Can you work these out from the model? Positions are in its coordinate system, mm. Give positions to 0.01 mm unless a question says otherwise; leave off trailing zeros. Write each loop counter-clockwise with the first axis right and the second up, starting at its lowest first coordinate (ties: lowest second). Pieces come first, ordered by that corner, then holes. Notation, with made-up numbers: (-11.5, 49) -> (45.5, 49) arc R27 cw to (45.5, 72) -> close; hole circle Ø4 at (-21.75, 54). An arc over 180 degrees is marked (long way). One line per item, written item: value.
from build123d import *

# Parameters (mm, degrees)
F0_W     = 508
F0_H     = 127
F0_R     = 9.525
F1_DEPTH = 25.4
F3_DEPTH = 101.6


# Not quite as in the source:
# - a fillet or chamfer that OpenCascade refuses, or shapes differently, is made with other operations: its cross-section is extruded or revolved along the edge and cut away or added


with BuildPart() as f1:
    # F0 (on Top) → F1 (new body)
    with BuildSketch(Plane.XY):
        with Locations((254, 63.5)):
            Rectangle(F0_W, F0_H)
        with Locations((63.5, 50.8)):
            Circle(F0_R, mode=Mode.SUBTRACT)
        with Locations((190.5, 50.8)):
            Circle(F0_R, mode=Mode.SUBTRACT)
        with Locations((317.5, 50.8)):
            Circle(F0_R, mode=Mode.SUBTRACT)
        with Locations((444.5, 50.8)):
            Circle(F0_R, mode=Mode.SUBTRACT)
        with Locations((63.5, 76.2)):
            Circle(F0_R, mode=Mode.SUBTRACT)
        with Locations((190.5, 76.2)):
            Circle(F0_R, mode=Mode.SUBTRACT)
        with Locations((317.5, 76.2)):
            Circle(F0_R, mode=Mode.SUBTRACT)
        with Locations((444.5, 76.2)):
            Circle(F0_R, mode=Mode.SUBTRACT)
    extrude(amount=F1_DEPTH)

    # F2: fillet of radius 5.08 on 16 edges, made by hand

    # F2_s1 → F2_t2 (revolve, cut)
    with BuildSketch(Plane.XZ.offset(-76.2)):
        with BuildLine():
            ThreePointArc((200.025, 20.32), (201.5128975516, 23.9121024484), (205.105, 25.4))
            Line((205.105, 25.4), (200.025, 25.4))
            Line((200.025, 25.4), (200.025, 20.32))
        make_face()
    revolve(axis=Axis((190.5, 76.2, 25.4), (0, 0, 1)), mode=Mode.SUBTRACT)

    # F2_s3 → F2_t4 (revolve, cut)
    with BuildSketch(Plane.XZ.offset(-50.8)):
        with BuildLine():
            ThreePointArc((200.025, 20.32), (201.5128975516, 23.9121024484), (205.105, 25.4))
            Line((205.105, 25.4), (200.025, 25.4))
            Line((200.025, 25.4), (200.025, 20.32))
        make_face()
    revolve(axis=Axis((190.5, 50.8, 25.4), (0, 0, 1)), mode=Mode.SUBTRACT)

    # F2_s5 → F2_t6 (revolve, cut)
    with BuildSketch(Plane.XZ.offset(-76.2)):
        with BuildLine():
            ThreePointArc((327.025, 20.32), (328.5128975516, 23.9121024484), (332.105, 25.4))
            Line((332.105, 25.4), (327.025, 25.4))
            Line((327.025, 25.4), (327.025, 20.32))
        make_face()
    revolve(axis=Axis((317.5, 76.2, 25.4), (0, 0, 1)), mode=Mode.SUBTRACT)

    # F2_s7 → F2_t8 (revolve, cut)
    with BuildSketch(Plane.XZ.offset(-50.8)):
        with BuildLine():
            ThreePointArc((327.025, 20.32), (328.5128975516, 23.9121024484), (332.105, 25.4))
            Line((332.105, 25.4), (327.025, 25.4))
            Line((327.025, 25.4), (327.025, 20.32))
        make_face()
    revolve(axis=Axis((317.5, 50.8, 25.4), (0, 0, 1)), mode=Mode.SUBTRACT)

    # F2_s9 → F2_t10 (revolve, cut)
    with BuildSketch(Plane.XZ.offset(-76.2)):
        with BuildLine():
            ThreePointArc((73.025, 20.32), (74.5128975516, 23.9121024484), (78.105, 25.4))
            Line((78.105, 25.4), (73.025, 25.4))
            Line((73.025, 25.4), (73.025, 20.32))
        make_face()
    revolve(axis=Axis((63.5, 76.2, 25.4), (0, 0, 1)), mode=Mode.SUBTRACT)

    # F2_s11 → F2_t12 (revolve, cut)
    with BuildSketch(Plane.XZ.offset(-50.8)):
        with BuildLine():
            ThreePointArc((73.025, 20.32), (74.5128975516, 23.9121024484), (78.105, 25.4))
            Line((78.105, 25.4), (73.025, 25.4))
            Line((73.025, 25.4), (73.025, 20.32))
        make_face()
    revolve(axis=Axis((63.5, 50.8, 25.4), (0, 0, 1)), mode=Mode.SUBTRACT)

    # F2_s13 → F2_t14 (revolve, cut)
    with BuildSketch(Plane.XZ.offset(-76.2)):
        with BuildLine():
            ThreePointArc((454.025, 20.32), (455.5128975516, 23.9121024484), (459.105, 25.4))
            Line((459.105, 25.4), (454.025, 25.4))
            Line((454.025, 25.4), (454.025, 20.32))
        make_face()
    revolve(axis=Axis((444.5, 76.2, 25.4), (0, 0, 1)), mode=Mode.SUBTRACT)

    # F2_s15 → F2_t16 (revolve, cut)
    with BuildSketch(Plane.XZ.offset(-50.8)):
        with BuildLine():
            ThreePointArc((454.025, 20.32), (455.5128975516, 23.9121024484), (459.105, 25.4))
            Line((459.105, 25.4), (454.025, 25.4))
            Line((454.025, 25.4), (454.025, 20.32))
        make_face()
    revolve(axis=Axis((444.5, 50.8, 25.4), (0, 0, 1)), mode=Mode.SUBTRACT)

    # F2_s17 → F2_t18 (revolve, cut)
    with BuildSketch(Plane.XZ.offset(-50.8)):
        with BuildLine():
            ThreePointArc((200.025, 5.08), (201.5128975516, 1.4878975516), (205.105, 0))
            Line((205.105, 0), (200.025, 0))
            Line((200.025, 0), (200.025, 5.08))
        make_face()
    revolve(axis=Axis((190.5, 50.8, 0), (0, 0, 1)), mode=Mode.SUBTRACT)

    # F2_s19 → F2_t20 (revolve, cut)
    with BuildSketch(Plane.XZ.offset(-76.2)):
        with BuildLine():
            ThreePointArc((200.025, 5.08), (201.5128975516, 1.4878975516), (205.105, 0))
            Line((205.105, 0), (200.025, 0))
            Line((200.025, 0), (200.025, 5.08))
        make_face()
    revolve(axis=Axis((190.5, 76.2, 0), (0, 0, 1)), mode=Mode.SUBTRACT)

    # F2_s21 → F2_t22 (revolve, cut)
    with BuildSketch(Plane.XZ.offset(-50.8)):
        with BuildLine():
            ThreePointArc((327.025, 5.08), (328.5128975516, 1.4878975516), (332.105, 0))
            Line((332.105, 0), (327.025, 0))
            Line((327.025, 0), (327.025, 5.08))
        make_face()
    revolve(axis=Axis((317.5, 50.8, 0), (0, 0, 1)), mode=Mode.SUBTRACT)

    # F2_s23 → F2_t24 (revolve, cut)
    with BuildSketch(Plane.XZ.offset(-76.2)):
        with BuildLine():
            ThreePointArc((327.025, 5.08), (328.5128975516, 1.4878975516), (332.105, 0))
            Line((332.105, 0), (327.025, 0))
            Line((327.025, 0), (327.025, 5.08))
        make_face()
    revolve(axis=Axis((317.5, 76.2, 0), (0, 0, 1)), mode=Mode.SUBTRACT)

    # F2_s25 → F2_t26 (revolve, cut)
    with BuildSketch(Plane.XZ.offset(-50.8)):
        with BuildLine():
            ThreePointArc((454.025, 5.08), (455.5128975516, 1.4878975516), (459.105, 0))
            Line((459.105, 0), (454.025, 0))
            Line((454.025, 0), (454.025, 5.08))
        make_face()
    revolve(axis=Axis((444.5, 50.8, 0), (0, 0, 1)), mode=Mode.SUBTRACT)

    # F2_s27 → F2_t28 (revolve, cut)
    with BuildSketch(Plane.XZ.offset(-76.2)):
        with BuildLine():
            ThreePointArc((454.025, 5.08), (455.5128975516, 1.4878975516), (459.105, 0))
            Line((459.105, 0), (454.025, 0))
            Line((454.025, 0), (454.025, 5.08))
        make_face()
    revolve(axis=Axis((444.5, 76.2, 0), (0, 0, 1)), mode=Mode.SUBTRACT)

    # F2_s29 → F2_t30 (revolve, cut)
    with BuildSketch(Plane.XZ.offset(-76.2)):
        with BuildLine():
            ThreePointArc((73.025, 5.08), (74.5128975516, 1.4878975516), (78.105, 0))
            Line((78.105, 0), (73.025, 0))
            Line((73.025, 0), (73.025, 5.08))
        make_face()
    revolve(axis=Axis((63.5, 76.2, 0), (0, 0, 1)), mode=Mode.SUBTRACT)

    # F2_s31 → F2_t32 (revolve, cut)
    with BuildSketch(Plane.XZ.offset(-50.8)):
        with BuildLine():
            ThreePointArc((73.025, 5.08), (74.5128975516, 1.4878975516), (78.105, 0))
            Line((78.105, 0), (73.025, 0))
            Line((73.025, 0), (73.025, 5.08))
        make_face()
    revolve(axis=Axis((63.5, 50.8, 0), (0, 0, 1)), mode=Mode.SUBTRACT)

    # F0 (on Top) → F3 (join)
    with BuildSketch(Plane.XY):
        with Locations((254, 63.5)):
            Rectangle(F0_W, F0_H)
        with Locations((63.5, 50.8)):
            Circle(F0_R, mode=Mode.SUBTRACT)
        with Locations((190.5, 50.8)):
            Circle(F0_R, mode=Mode.SUBTRACT)
        with Locations((317.5, 50.8)):
            Circle(F0_R, mode=Mode.SUBTRACT)
        with Locations((444.5, 50.8)):
            Circle(F0_R, mode=Mode.SUBTRACT)
        with Locations((63.5, 76.2)):
            Circle(F0_R, mode=Mode.SUBTRACT)
        with Locations((190.5, 76.2)):
            Circle(F0_R, mode=Mode.SUBTRACT)
        with Locations((317.5, 76.2)):
            Circle(F0_R, mode=Mode.SUBTRACT)
        with Locations((444.5, 76.2)):
            Circle(F0_R, mode=Mode.SUBTRACT)
    extrude(amount=F3_DEPTH)


solid = f1.part
1) If we section it at A-A (x = 190.5): Write out the boundary of the cut face in (y, z) (3 decimals).
Answer list:
outline: (0, 0) -> (41.275, 0) -> (41.275, 101.6) -> (0, 101.6) -> close; (60.325, 0) -> (66.675, 0) -> (66.675, 101.6) -> (60.325, 101.6) -> close; (85.725, 0) -> (127, 0) -> (127, 101.6) -> (85.725, 101.6) -> close
2) If we section it at B-B (z = 53): State how many separate pieces and enclosed holes the cut face has, and give its area (3 significant figures).
Answer list:
separate pieces: 1
enclosed holes: 8
area: 62,200 mm^2
3) If we section it at D-D (y = 55.5): Write out the boundary of the cut face in (x, z), and give its area (3 significant figures).
Answer list:
outline: (0, 0) -> (55.22, 0) -> (55.22, 101.6) -> (0, 101.6) -> close; (71.78, 0) -> (182.22, 0) -> (182.22, 101.6) -> (71.78, 101.6) -> close; (198.78, 0) -> (309.22, 0) -> (309.22, 101.6) -> (198.78, 101.6) -> close; (325.78, 0) -> (436.22, 0) -> (436.22, 101.6) -> (325.78, 101.6) -> close; (452.78, 0) -> (508, 0) -> (508, 101.6) -> (452.78, 101.6) -> close
area: 44,900 mm^2
4) We'd pull the mould along X, two halves only. Please class faces 1 (the face through (250, 0, 50)), 2 (the face through (434.984, 51.219, 50.089)), 3 (the face through (0, 63, 50)): released by +X, released by -X, zero draft, split by the parting line, or undercut.
Answer list:
face 1: zero draft
face 2: undercut
face 3: released by -X
5) If we section it at C-C (y = 76.2): Write out the boundary of the cut face in (x, z) (3 decimals), and give its area (3 significant figures).
Answer list:
outline: (0, 0) -> (53.975, 0) -> (53.975, 101.6) -> (0, 101.6) -> close; (73.025, 0) -> (180.975, 0) -> (180.975, 101.6) -> (73.025, 101.6) -> close; (200.025, 0) -> (307.975, 0) -> (307.975, 101.6) -> (200.025, 101.6) -> close; (327.025, 0) -> (434.975, 0) -> (434.975, 101.6) -> (327.025, 101.6) -> close; (454.025, 0) -> (508, 0) -> (508, 101.6) -> (454.025, 101.6) -> close
area: 43,900 mm^2
6) I need wall thicknesses on L1, parallel to X at y = 50, z = 57; L2, parallel to Y at x = 317, z = 26; L3, parallel to X at y = 81, z = 19. Which ranges of each line are inside material? Lowest first, please.
Answer list:
L1: x = 0 to 54.01, 72.99 to 181.01, 199.99 to 308.01, 326.99 to 435.01, 453.99 to 508
L2: y = 0 to 41.29, 60.31 to 66.69, 85.71 to 127
L3: x = 0 to 55.27, 71.73 to 182.27, 198.73 to 309.27, 325.73 to 436.27, 452.73 to 508
